```python
from build123d import *

# Parameters (mm, degrees)
SKETCH1_W           = 40
SKETCH1_H           = 27
SKETCH1_W_2         = 32
SKETCH1_H_2         = 7
BOSS_EXTRUDE1_DEPTH = 5
SKETCH1_3_W         = 32
SKETCH1_3_H         = 7
BOSS_EXTRUDE2_DEPTH = 45
CUT_EXTRUDE1_REACH  = 54.096
SKETCH2_R           = 8.7757
CUT_EXTRUDE2_REACH  = 54.096
SKETCH4_R           = 1.7
CUT_EXTRUDE3_REACH  = 48.715
SKETCH5_R           = 1.7
CUT_EXTRUDE5_REACH  = 48.715
SKETCH7_W           = 40
SKETCH7_H           = 10
SKETCH8_R           = 1.7
CUT_EXTRUDE6_DEPTH  = 6.35


with BuildPart() as part:
    # Sketch1 → Boss-Extrude1 (new body)
    with BuildSketch(Plane(origin=(0, 0, 0), x_dir=(1, 0, 0), z_dir=(0, 1, 0))):
        Rectangle(SKETCH1_W, SKETCH1_H)
        Rectangle(SKETCH1_W_2, SKETCH1_H_2, mode=Mode.SUBTRACT)
    extrude(amount=BOSS_EXTRUDE1_DEPTH)

    # Sketch1_3 → Boss-Extrude2 (add)
    with BuildSketch(Plane(origin=(0, 0, 0), x_dir=(1, 0, 0), z_dir=(0, 1, 0))):
        Rectangle(SKETCH1_3_W, SKETCH1_3_H)
    extrude(amount=BOSS_EXTRUDE2_DEPTH)

    # Sketch2 → Cut-Extrude1 (cut, up to next)
    with BuildSketch(Plane.XY.offset(3.5), mode=Mode.PRIVATE) as cut_extrude1_sk1:
        with Locations((0, 28.5)):
            Circle(SKETCH2_R)
    cut_extrude1_tool1 = extrude(cut_extrude1_sk1.sketch, amount=-CUT_EXTRUDE1_REACH, mode=Mode.PRIVATE) & part.part
    add(cut_extrude1_tool1.solids().sort_by_distance((0, 28.5, 3.5))[0], mode=Mode.SUBTRACT)

    # Sketch4 → Cut-Extrude2 (cut, up to next)
    with BuildSketch(Plane.XY.offset(3.5), mode=Mode.PRIVATE) as cut_extrude2_sk1:
        with Locations((0, 41.2)):
            Circle(SKETCH4_R)
    cut_extrude2_tool1 = extrude(cut_extrude2_sk1.sketch, amount=-CUT_EXTRUDE2_REACH, mode=Mode.PRIVATE) & part.part
    # Sketch4 → Cut-Extrude2 (cut, up to next)
    with BuildSketch(Plane.XY.offset(3.5), mode=Mode.PRIVATE) as cut_extrude2_sk2:
        with Locations((12.7, 28.5)):
            Circle(SKETCH4_R)
    cut_extrude2_tool2 = extrude(cut_extrude2_sk2.sketch, amount=-CUT_EXTRUDE2_REACH, mode=Mode.PRIVATE) & part.part
    # Sketch4 → Cut-Extrude2 (cut, up to next)
    with BuildSketch(Plane.XY.offset(3.5), mode=Mode.PRIVATE) as cut_extrude2_sk3:
        with Locations((0, 15.8)):
            Circle(SKETCH4_R)
    cut_extrude2_tool3 = extrude(cut_extrude2_sk3.sketch, amount=-CUT_EXTRUDE2_REACH, mode=Mode.PRIVATE) & part.part
    # Sketch4 → Cut-Extrude2 (cut, up to next)
    with BuildSketch(Plane.XY.offset(3.5), mode=Mode.PRIVATE) as cut_extrude2_sk4:
        with Locations((-12.7, 28.5)):
            Circle(SKETCH4_R)
    cut_extrude2_tool4 = extrude(cut_extrude2_sk4.sketch, amount=-CUT_EXTRUDE2_REACH, mode=Mode.PRIVATE) & part.part
    add(cut_extrude2_tool1.solids().sort_by_distance((0, 41.2, 3.5))[0], mode=Mode.SUBTRACT)
    add(cut_extrude2_tool2.solids().sort_by_distance((12.7, 28.5, 3.5))[0], mode=Mode.SUBTRACT)
    add(cut_extrude2_tool3.solids().sort_by_distance((0, 15.8, 3.5))[0], mode=Mode.SUBTRACT)
    add(cut_extrude2_tool4.solids().sort_by_distance((-12.7, 28.5, 3.5))[0], mode=Mode.SUBTRACT)

    # Sketch5 → Cut-Extrude3 (cut, up to next)
    with BuildSketch(Plane(origin=(0, 5, 0), x_dir=(1, 0, 0), z_dir=(0, 1, 0)), mode=Mode.PRIVATE) as cut_extrude3_sk1:
        with Locations(Location((-16.5, 10, 0), (0, 0, 270))):
            Circle(SKETCH5_R)
    cut_extrude3_tool1 = extrude(cut_extrude3_sk1.sketch, amount=-CUT_EXTRUDE3_REACH, mode=Mode.PRIVATE) & part.part
    # Sketch5 → Cut-Extrude3 (cut, up to next)
    with BuildSketch(Plane(origin=(0, 5, 0), x_dir=(1, 0, 0), z_dir=(0, 1, 0)), mode=Mode.PRIVATE) as cut_extrude3_sk2:
        with Locations(Location((-16.5, -10, 0), (0, 0, 270))):
            Circle(SKETCH5_R)
    cut_extrude3_tool2 = extrude(cut_extrude3_sk2.sketch, amount=-CUT_EXTRUDE3_REACH, mode=Mode.PRIVATE) & part.part
    # Sketch5 → Cut-Extrude3 (cut, up to next)
    with BuildSketch(Plane(origin=(0, 5, 0), x_dir=(1, 0, 0), z_dir=(0, 1, 0)), mode=Mode.PRIVATE) as cut_extrude3_sk3:
        with Locations(Location((16.5, -10, 0), (0, 0, 90))):
            Circle(SKETCH5_R)
    cut_extrude3_tool3 = extrude(cut_extrude3_sk3.sketch, amount=-CUT_EXTRUDE3_REACH, mode=Mode.PRIVATE) & part.part
    # Sketch5 → Cut-Extrude3 (cut, up to next)
    with BuildSketch(Plane(origin=(0, 5, 0), x_dir=(1, 0, 0), z_dir=(0, 1, 0)), mode=Mode.PRIVATE) as cut_extrude3_sk4:
        with Locations(Location((16.5, 10, 0), (0, 0, 90))):
            Circle(SKETCH5_R)
    cut_extrude3_tool4 = extrude(cut_extrude3_sk4.sketch, amount=-CUT_EXTRUDE3_REACH, mode=Mode.PRIVATE) & part.part
    add(cut_extrude3_tool1.solids().sort_by_distance((-16.5, 5, -10))[0], mode=Mode.SUBTRACT)
    add(cut_extrude3_tool2.solids().sort_by_distance((-16.5, 5, 10))[0], mode=Mode.SUBTRACT)
    add(cut_extrude3_tool3.solids().sort_by_distance((16.5, 5, 10))[0], mode=Mode.SUBTRACT)
    add(cut_extrude3_tool4.solids().sort_by_distance((16.5, 5, -10))[0], mode=Mode.SUBTRACT)

    # Sketch7 → Cut-Extrude5 (cut, up to next)
    with BuildSketch(Plane(origin=(0, 5, 0), x_dir=(1, 0, 0), z_dir=(0, 1, 0)), mode=Mode.PRIVATE) as cut_extrude5_sk1:
        with Locations((0, 8.5)):
            Rectangle(SKETCH7_W, SKETCH7_H)
    cut_extrude5_tool1 = extrude(cut_extrude5_sk1.sketch, amount=-CUT_EXTRUDE5_REACH, mode=Mode.PRIVATE) & part.part
    add(cut_extrude5_tool1.solids().sort_by_distance((0, 5, -8.5))[0], mode=Mode.SUBTRACT)

    # Sketch8 → Cut-Extrude6 (cut)
    with BuildSketch(Plane(origin=(0, 0, -3.5), x_dir=(-1, 0, 0), z_dir=(0, 0, -1))):
        with Locations((-12.7, 2.5)):
            Circle(SKETCH8_R)
        with Locations(Location((12.7, 2.5, 0), (0, 0, 180))):
            Circle(SKETCH8_R)
    extrude(amount=-CUT_EXTRUDE6_DEPTH, mode=Mode.SUBTRACT)


solid = part.part
```
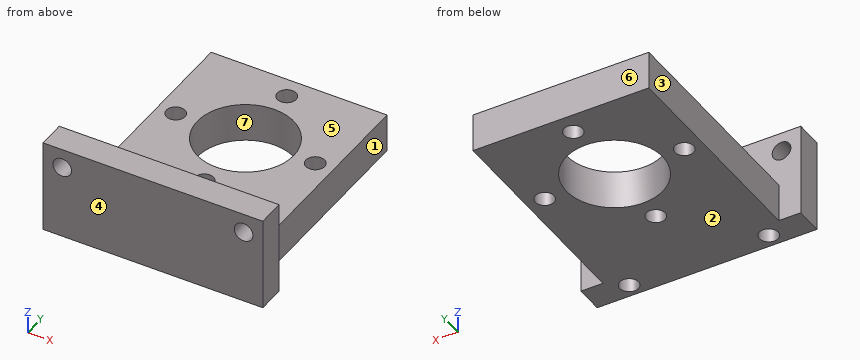
Verification items for the finished model (mm, model axes). Face numbers are marked on the shaded views. A direction names the side the tool comes from. Coordinates: 2 decimals unless noted, no trailing zeros. Loops run counter-clockwise (first coordinate to the right, second up) from the corner with the lowest first, then second, coordinate; pieces in that order, holes last. Notation, with made-up numbers: (-3, 16) - (53, 16) arc R23 cw to (53, 27) - close; hole circle Ø4 at (-18, 11.5). An arc over 180 degrees is marked (long way). Return JSON: item names as keys, results as strings.
1. Section check D-D, the plane x = 12.7. Record the boundary of the cut face in (y, z), then the cut area to 3 significant figures.
Established:
{"outline": "(0, -3.5) - (0.8, -3.5) - (0.8, 2.85) - (4.2, 2.85) - (4.2, -3.5) - (26.8, -3.5) - (26.8, 3.5) - (5, 3.5) - (5, 13.5) - (0, 13.5) - close; (30.2, -3.5) - (45, -3.5) - (45, 3.5) - (30.2, 3.5) - close", "area": "320 mm2"}
2. Section check A-A, the plane y = 15.8. Record the boundary of the cut face in (x, z).
Established:
{"outline": "(-16, -3.5) - (-1.7, -3.5) - (-1.7, 3.5) - (-16, 3.5) - close; (1.7, -3.5) - (16, -3.5) - (16, 3.5) - (1.7, 3.5) - close"}
3. Section check C-C, the plane y = 28.5. Record the boundary of the cut face in (x, z), then the cut area to 3 significant figures.
Established:
{"outline": "(-16, -3.5) - (-14.4, -3.5) - (-14.4, 3.5) - (-16, 3.5) - close; (-11, -3.5) - (-8.78, -3.5) - (-8.78, 3.5) - (-11, 3.5) - close; (8.78, -3.5) - (11, -3.5) - (11, 3.5) - (8.78, 3.5) - close; (14.4, -3.5) - (16, -3.5) - (16, 3.5) - (14.4, 3.5) - close", "area": "53.5 mm2"}
4. Go/stop test with flat-tipped pins: pin 1 (10 mm diameter, centred on x = 15.5, y = 39.5, fed in from +Z); pin 2 (1 mm diameter, centred on x = 13.5, y = 3, fed in from -Z); pin 3 (2 mm diameter, centred on x = 16.5, z = 10, fed in from -Y); pin 4 (3.5 mm diameter, centred on y = 29, z = 1.5, fed in from -X). Record where each tip stops, or that it passes through.
Established:
{"pin 1": "stops at z = 3.5", "pin 2": "stops at z = 2.85", "pin 3": "passes through", "pin 4": "stops at x = -16"}
5. Thickness scan on L1, parallel to Y at x = 12.7, z = -0.75; L2, parallel to X at y = 2.55, z = 10; L3, parallel to Y at x = 12, z = -2.5. Record the ranges inside material, lowest first.
Established:
{"L1": "y = 0 to 0.8, 4.2 to 26.8, 30.2 to 45", "L2": "x = -20 to -18.2, -14.8 to 14.8, 18.2 to 20", "L3": "y = 0 to 0.95, 4.05 to 26.95, 30.05 to 45"}
6. Section check B-B, the plane x = 0. Record the boundary of the cut face in (y, z).
Established:
{"outline": "(0, -3.5) - (14.1, -3.5) - (14.1, 3.5) - (5, 3.5) - (5, 13.5) - (0, 13.5) - close; (17.5, -3.5) - (19.72, -3.5) - (19.72, 3.5) - (17.5, 3.5) - close; (37.28, -3.5) - (39.5, -3.5) - (39.5, 3.5) - (37.28, 3.5) - close; (42.9, -3.5) - (45, -3.5) - (45, 3.5) - (42.9, 3.5) - close"}
7. Mould release check, pull along Y, two halves, no side actions. Record for the marked faces 4, 5, 6 and 7: +Y half, -Y half, draft (parallel to the pull), parting line (faces both ways), or undercut.
Established:
{"face 4": "-Y half", "face 5": "draft", "face 6": "+Y half", "face 7": "undercut"}
8. Tool access check on the marked faces 1, 2 and 3. Record the directions out of +Z, -Z, +X, -X, +Y, -Y that give a thin tool (end or side, any length) a straight path to the whole face; none if there is none.
Established:
{"face 1": "+Z, -Z, +X, +Y", "face 2": "-Z, +X, -X, +Y, -Y", "face 3": "+Z, -Z, -X, +Y"}
